Work out the finished part from the listing and answer in its coordinate system (mm). Face numbers are marked on the shaded views. A direction names the side the tool comes from. Give positions to 0.01 mm unless a question says otherwise; leave off trailing zeros. Order: outer loops, then holes, each group sorted by start corner. A loop starts at its lowest first (then second) coordinate and runs counter-clockwise, first axis right, second up.
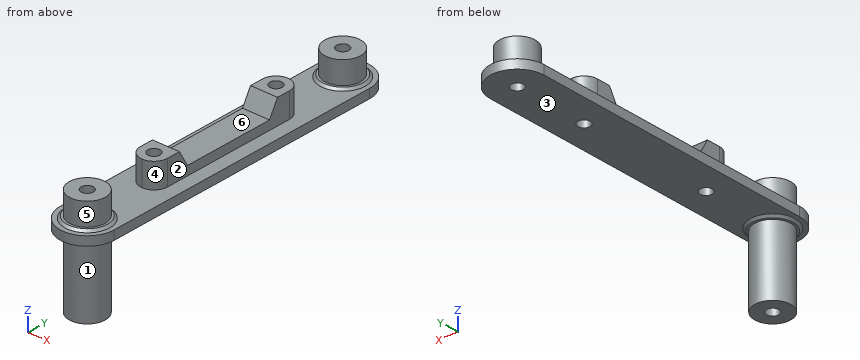
```python
from build123d import *

# Parameters (mm, degrees)
F1_DEPTH       = 3.175
F2_W           = 9.525
F2_H           = 58.0526056528
F2_R           = 6.35
F3_DEPTH       = 8.6995
F5_DEPTH       = 9.525
F6_R           = 4.76249
F7_R           = 6.35
F8_DEPTH       = 25.4
F9_R           = 2.15265
F10_DEPTH      = 37.2745
F11_R          = 7.14375
F11_R_2        = 2.15265
F12_DEPTH      = 0.79375
F12_DEPTH_BACK = 3.96875
F13_R          = 7.14375
F13_R_2        = 2.15265
F14_DEPTH      = 0.79375
F15_SIZE       = 0.79374


# Not quite as in the source:
# - a fillet or chamfer is up to 0.001 mm smaller than in the source, because OpenCascade refuses the exact size


with BuildPart() as f1:
    # F0 (on Top) → F1 (new body)
    with BuildSketch(Plane.XY):
        with BuildLine():
            Line((0, 101.6), (0, 0))
            ThreePointArc((0, 0), (9.525, -9.525), (19.05, 0))
            Line((19.05, 0), (19.05, 101.6))
            ThreePointArc((19.05, 101.6), (9.525, 111.125), (0, 101.6))
        make_face()
    extrude(amount=F1_DEPTH)

    # F2 (on face) → F3 (join)
    with BuildSketch(Plane.XY.offset(3.175)):
        with Locations((9.525, 50.8)):
            Rectangle(F2_W, F2_H)
        with Locations((9.525, 0)):
            Circle(F2_R)
        with Locations((9.525, 101.6)):
            Circle(F2_R)
    extrude(amount=F3_DEPTH)

    # F4 (on face) → F5 (cut, through all)
    with BuildSketch(Plane(origin=(4.7625, 0, 0), x_dir=(0, -1, 0), z_dir=(-1, 0, 0))):
        Polygon((-34.4882687357, 6.35), (-31.2986971736, 11.8745), (-70.3013028264, 11.8745), (-67.1117312643, 6.35), align=None)
    extrude(amount=-F5_DEPTH, mode=Mode.SUBTRACT)

    # F6 (radius 4.7625 in the source; OpenCascade refuses exactly that, so slightly less here)
    f6_edges = [f1.edges().sort_by_distance(p)[0] for p in [
        (4.7625, 79.826303, 7.52475),
        (14.2875, 79.826303, 7.52475),
        (4.7625, 21.773697, 7.52475),
        (14.2875, 21.773697, 7.52475),
    ]]
    fillet(f6_edges, radius=F6_R)

    # F7 (on face) → F8 (join)
    with BuildSketch(Plane(origin=(0, 0, 0), x_dir=(1, 0, 0), z_dir=(0, 0, -1))):
        with Locations((9.525, 0)):
            Circle(F7_R)
    extrude(amount=F8_DEPTH)

    # F9 (on face) → F10 (cut, through all)
    with BuildSketch(Plane(origin=(0, 0, -25.4), x_dir=(1, 0, 0), z_dir=(0, 0, -1))):
        with Locations((9.525, 0)):
            Circle(F9_R)
        with Locations((9.525, -26.5361971736)):
            Circle(F9_R)
        with Locations((9.525, -75.0638028264)):
            Circle(F9_R)
        with Locations((9.525, -101.6)):
            Circle(F9_R)
    extrude(amount=-F10_DEPTH, mode=Mode.SUBTRACT)

    # F11 (on face) → F12 (join, two sides)
    with BuildSketch(Plane.XY.offset(3.175)) as f12_sk:
        with Locations((9.525, 0)):
            Circle(F11_R)
        with Locations((9.525, 0)):
            Circle(F11_R_2, mode=Mode.SUBTRACT)
    extrude(amount=F12_DEPTH)
    extrude(f12_sk.sketch, amount=-F12_DEPTH_BACK)

    # F13 (on face) → F14 (join, through all)
    with BuildSketch(Plane.XY.offset(3.175)):
        with Locations((9.525, 101.6)):
            Circle(F13_R)
        with Locations((9.525, 101.6)):
            Circle(F13_R_2, mode=Mode.SUBTRACT)
    extrude(amount=F14_DEPTH)

    # F15 (size 0.79375 in the source; OpenCascade refuses exactly that, so slightly less here)
    f15_edges = [f1.edges().sort_by_distance(p)[0] for p in [
        (2.38125, 101.6, 3.175),
        (2.38125, 0, 0),
        (2.38125, 0, 3.175),
    ]]
    chamfer(f15_edges, length=F15_SIZE)


solid = f1.part
```
1. Straight lines are drawn through the part: probe 1 along Z at (x, y) = (15.25, 22) (3 decimals); probe 2 along X at (y, z) = (101, 5); probe 3 along Z at (x, y) = (9.25, 56). For each, find the intervals that lie inside material, in ascending order.
Findings below:
probe 1: z = 0 to 3.175
probe 2: x = 3.2 to 7.46, 11.59 to 15.85
probe 3: z = 0 to 6.35
2. Which of the six approach directions +Z, -Z, +X, -X, +Y, -Y give full straight-line access (tool end or side, diameter ignored) to the marked faces 4, 5 and 6?
Findings below:
face 4: +Z, +X
face 5: +Z
face 6: +Z, +X, -X
3. The mould has two halves that part along Y. Classify the marked faces 1, 2 and 3: pulls with the +Y half, pulls with the -Y half, needs draft (parallel to the pull), parting line crosses it, or undercut.
Findings below:
face 1: parting line crosses it
face 2: undercut
face 3: needs draft
4. The part is cut by section A-A (z = -12). Write down the section's boundary in (x, y) (3 decimals), then the cut area to 3 significant figures.
Findings below:
outline: circle Ø12.7 at (9.525, 0); hole circle Ø4.305 at (9.525, 0)
area: 112 mm2
5. Given P1, Ø3, axis at x = 5.5, y = 88, coming from the +Z side (3 decimals); P2, Ø4, axis at x = 6.5, y = 39, coming from the -Z side; P3, Ø3, axis at x = 14.5, z = -1, coming from the -Y side, each flat-ended and moving along its own axis, determine where each tip first touches the part or whether it passes through.
Findings below:
P1: stops at z = 3.175
P2: stops at z = 0
P3: stops at y = -8.71
